from build123d import *

# Parameters (mm, degrees)
BOSS_EXTRUDE3_DEPTH = 10
FILLET1_R           = 10
FILLET2_R           = 10
FILLET3_R           = 10
FILLET4_R           = 70
FILLET5_R           = 70
BOSS_EXTRUDE5_START = -10
BOSS_EXTRUDE5_DEPTH = 10
CUT_EXTRUDE1_REACH  = 123.684
SKETCH4_W           = 10
SKETCH4_H           = 7.527652991


with BuildPart() as part:
    # Sketch1 → Boss-Extrude3 (new body)
    with BuildSketch(Plane.XY):
        with BuildLine():
            Line((-76.083611013, -33.881828403), (45.731586831, -33.881828403))
            ThreePointArc((45.731586831, -33.881828403), (66.105293747, -14.631662941), (48.04052972, 6.80011497))
            Line((48.04052972, 6.80011497), (-43.429508159, 44.774039787))
            Line((-43.429508159, 44.774039787), (-76.083611013, -33.881828403))
        make_face()
        with BuildLine():
            Line((-61.104581002, -23.881828403), (45.731586831, -23.881828403))
            ThreePointArc((45.731586831, -23.881828403), (56.138081657, -13.475333577), (45.731586831, -3.068838752))
            Line((45.731586831, -3.068838752), (-38.028005668, 31.704082983))
            Line((-38.028005668, 31.704082983), (-61.104581002, -23.881828403))
        make_face(mode=Mode.SUBTRACT)
    extrude(amount=BOSS_EXTRUDE3_DEPTH)

    # Fillet1
    fillet1_edges = [part.edges().sort_by_distance(p)[0] for p in [
        (-76.083611013, -33.881828403, 5),
    ]]
    fillet(fillet1_edges, radius=FILLET1_R)

    # Fillet2
    fillet2_edges = [part.edges().sort_by_distance(p)[0] for p in [
        (-61.104581002, -23.881828403, 5),
    ]]
    fillet(fillet2_edges, radius=FILLET2_R)

    # Fillet3
    fillet3_edges = [part.edges().sort_by_distance(p)[0] for p in [
        (-38.028005668, 31.704082983, 5),
        (-43.429508159, 44.774039787, 5),
    ]]
    fillet(fillet3_edges, radius=FILLET3_R)

    # Fillet4
    fillet4_edges = [part.edges().sort_by_distance(p)[0] for p in [
        (48.04052972, 6.80011497, 5),
    ]]
    fillet(fillet4_edges, radius=FILLET4_R)

    # Fillet5
    fillet5_edges = [part.edges().sort_by_distance(p)[0] for p in [
        (45.731586831, -3.068838752, 5),
    ]]
    fillet(fillet5_edges, radius=FILLET5_R)

    # Sketch3 → Boss-Extrude5 (add)
    with BuildSketch(Plane.XY.offset(10).offset(BOSS_EXTRUDE5_START)):
        with BuildLine():
            Line((-61.104581002, -33.881828403), (45.731586831, -33.881828403))
            ThreePointArc((45.731586831, -33.881828403), (49.984539158, -33.433725987), (54.050711911, -32.109098334))
            ThreePointArc((54.050711911, -32.109098334), (54.926134679, -38.48550442), (54.050711911, -44.861910507))
            Line((54.050711911, -44.861910507), (41.297899737, -44.861910507))
            Line((41.297899737, -44.861910507), (-65.538268096, -44.861910507))
            Line((-65.538268096, -44.861910507), (-61.104581002, -33.881828403))
        make_face()
        with BuildLine():
            Line((-59.755272984, -35.881828403), (45.731586831, -35.881828403))
            ThreePointArc((45.731586831, -35.881828403), (49.213208875, -35.609680605), (52.610255818, -34.799848187))
            ThreePointArc((52.610255818, -34.799848187), (52.923282115, -38.83702206), (52.47940001, -42.861910507))
            Line((52.47940001, -42.861910507), (41.297899737, -42.861910507))
            Line((41.297899737, -42.861910507), (-62.5737856, -42.861910507))
            Line((-62.5737856, -42.861910507), (-59.755272984, -35.881828403))
        make_face(mode=Mode.SUBTRACT)
    extrude(amount=BOSS_EXTRUDE5_DEPTH)

    # Sketch4 → Cut-Extrude1 (cut, up to next)
    with BuildSketch(Plane(origin=(-38.920465473, 15.715835623, 0), x_dir=(0, 0, -1), z_dir=(0.9272587501851874, -0.37442116687629234, 0)), mode=Mode.PRIVATE) as cut_extrude1_sk1:
        with Locations((-5, -59.409204893)):
            Rectangle(SKETCH4_W, SKETCH4_H)
    cut_extrude1_tool1 = extrude(cut_extrude1_sk1.sketch, amount=-CUT_EXTRUDE1_REACH, mode=Mode.PRIVATE) & part.part
    add(cut_extrude1_tool1.solids().sort_by_distance((-61.164529, -39.371869, 5))[0], mode=Mode.SUBTRACT)


solid = part.part
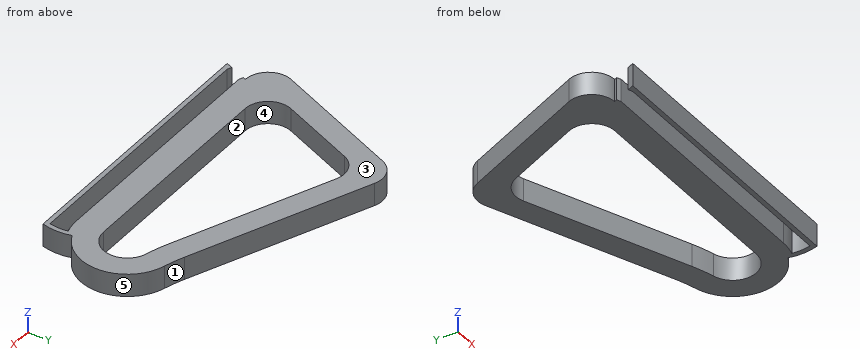
Verification items for the finished model (mm, model axes). Face numbers are marked on the shaded views. A direction names the side the tool comes from. Give positions to 0.01 mm unless a question says otherwise; leave off trailing zeros. Loops run counter-clockwise (first coordinate to the right, second up) from the corner with the lowest first, then second, coordinate; pieces in that order, holes last. Notation, with made-up numbers: (-25, 46) - (4, 46) arc R34 cw to (4, 78) - close; hole circle Ø3 at (50, 45). An arc over 180 degrees is marked (long way). Write item = value, one per line. Start each with the question number.
Q1. Cross-section at B-B, the plane x = 14. Enter the section's corners in (y, z).
Q2. Tool access check on the marked faces 1 and 2. Record the directions out of +Z, -Z, +X, -X, +Y, -Y that give a thin tool (end or side, any length) a straight path to the whole face; none if there is none.
Q3. Thickness scan on line 1 (Y direction, x = -1, z = 4); line 2 (Y direction, x = 45.5, z = 8.5); line 3 (X direction, y = -15.5, z = 5). Record the ranges inside material, lowest first.
Q4. Cross-section at D-D, the plane y = -7.5. Enter the section's corners in (x, z), and give its area (3 significant figures).
Q5. Cross-section at A-A, the plane z = 8. Enter the section's corners in (x, y).
Q6. Depth check by flat-ended pin: P1, Ø1, axis at y = -19, z = 5.5, coming from the +X side; P2, Ø5, axis at x = -5.5, z = 3, coming from the +Y side; P3, Ø1, axis at x = -0.5, z = 3, coming from the +Y side. Enter the tip coordinate at first touch or a pass-through.
Q7. Mould release check, pull along X, two halves, no side actions. Record for the marked faces 3, 4 and 5: released by +X, released by -X, zero draft, split by the parting line, or undercut.
Q8. Cross-section at C-C, the plane y = 18.5. Enter the section's corners in (x, z), and give its area (3 significant figures).
Answer key:
q1.outline = (-44.86, 0) - (-42.86, 0) - (-42.86, 10) - (-44.86, 10) - close; (-35.88, 0) - (-23.88, 0) - (-23.88, 10) - (-35.88, 10) - close; (10.1, 0) - (20.93, 0) - (20.93, 10) - (10.1, 10) - close
q2.face_1 = +Z, -Z, +X, +Y
q2.face_2 = +Z, -Z
q3.line_1 = -44.86 to -42.86, -35.88 to -23.88, 16.33 to 27.16
q3.line_2 = -44.86 to -42.86, -35.88 to -23.88, -2.6 to 7.95
q3.line_3 = -68.45 to -55.99, 55.94 to 66.04
q4.outline = (-65.13, 0) - (-54.3, 0) - (-54.3, 10) - (-65.13, 10) - close; (54.25, 0) - (65.24, 0) - (65.24, 10) - (54.25, 10) - close
q4.area = 218 mm^2
q5.outline = (-70.34, -20.05) arc R10 ccw to (-61.1, -33.88) - (-61.61, -35.13) - (-59.76, -35.88) - (45.73, -35.88) arc R22.41 ccw to (52.61, -34.8) arc R21.66 cw to (52.48, -42.86) - (-62.57, -42.86) - (-64.43, -42.11) - (-65.54, -44.86) - (54.05, -44.86) arc R23.66 ccw to (54.05, -32.11) arc R20.41 ccw to (50.99, 6.24) arc R70 cw to (42.2, 9.22) - (-34.19, 40.94) arc R10 ccw to (-47.26, 35.54) - close; hole (-55.36, -10.05) arc R10 ccw to (-46.13, -23.88) - (45.73, -23.88) arc R10.41 ccw to (48.33, -3.4) arc R70 cw to (39, -0.27) - (-28.79, 27.87) arc R10 ccw to (-41.86, 22.47) - close
q6.P1 = 65.51
q6.P2 = 30.07
q6.P3 = 27.16
q7.face_3 = zero draft
q7.face_4 = undercut
q7.face_5 = released by +X
q8.outline = (-54.34, 0) - (-43.51, 0) - (-43.51, 10) - (-54.34, 10) - close; (-6.22, 0) - (19.86, 0) - (19.86, 10) - (-6.22, 10) - close
q8.area = 369 mm^2
